from build123d import *

# Parameters (mm, degrees)
F0_W     = 76.2
F0_H     = 101.6
F1_DEPTH = 50.8
F2_W     = 101.6
F2_H     = 330
F3_DEPTH = 12.7
F4_W     = 101.6
F4_H     = 10
F5_DEPTH = 25.4
F6_W     = 63.5
F6_H     = 88.9
F7_DEPTH = 44.45
F9_DEPTH = 114.808


with BuildPart() as f1:
    # F0 (on Top) → F1 (new body)
    with BuildSketch(Plane.XY):
        Rectangle(F0_W, F0_H)
    extrude(amount=F1_DEPTH)

    # F2 (on face) → F3 (join)
    with BuildSketch(Plane.YZ.offset(38.1)):
        with Locations((0, 165)):
            Rectangle(F2_W, F2_H)
    extrude(amount=-F3_DEPTH)

    # F4 (on face) → F5 (join)
    with BuildSketch(Plane.YZ.offset(38.1)):
        with Locations((0, 325)):
            Rectangle(F4_W, F4_H)
        with Locations((0, 213.4)):
            Rectangle(F4_W, F4_H)
    extrude(amount=F5_DEPTH)

    # F6 (on face) → F7 (cut)
    with BuildSketch(Plane(origin=(0, 0, 0), x_dir=(1, 0, 0), z_dir=(0, 0, -1))):
        Rectangle(F6_W, F6_H)
    extrude(amount=-F7_DEPTH, mode=Mode.SUBTRACT)

    # F8 (on face) → F9 (cut)
    with BuildSketch(Plane.XZ.offset(50.8)):
        with BuildLine():
            ThreePointArc((-27.784303, 0), (-5.013912, -1.01281), (6.673748, 18.555406))
            ThreePointArc((6.673748, 18.555406), (0.164196, 34.270854), (-15.551252, 40.780406))
            ThreePointArc((-15.551252, 40.780406), (-36.839095, 24.9412), (-27.784303, 0))
        make_face()
        with BuildLine():
            ThreePointArc((-27.784303, 0), (-36.839095, 24.9412), (-15.551252, 40.780406))
            Line((-15.551252, 40.780406), (-38.1, 40.780406))
            Line((-38.1, 40.780406), (-38.1, 0))
            Line((-38.1, 0), (-27.784303, 0))
        make_face()
    extrude(amount=-F9_DEPTH, mode=Mode.SUBTRACT)


solid = f1.part
The model under review builds one solid part; all positions refer to its coordinate system, in mm. A direction names the side the tool comes from. Round coordinates to 2 decimals unless told otherwise and drop trailing zeros. Loops run counter-clockwise (first coordinate to the right, second up) from the corner with the lowest first, then second, coordinate; pieces in that order, holes last. Notation, with made-up numbers: (51.25, 73) -> (78.25, 73) arc R18 ccw to (78.25, 96) -> close; hole circle Ø8 at (-14, 55.25). An arc over 180 degrees is marked (long way). Return JSON: item names as keys, results as strings.
(1) Add section A-A on x = 45.5. Write out the cut boundary in (y, z), plus the area to 3 significant figures.
Solved:
{"outline": "(-50.8, 208.4) -> (50.8, 208.4) -> (50.8, 218.4) -> (-50.8, 218.4) -> close; (-50.8, 320) -> (50.8, 320) -> (50.8, 330) -> (-50.8, 330) -> close", "area": "2,030 mm2"}
(2) The part is to be moulded in two halves that separate along Z. For faces 1 (the flat face through (28, 50.8, 140)), 2 (the flat face through (38.1, -1, 268)), 3 (the flat face through (-33, -4, 40.78)), 4 (the flat face through (-7, 1, 50.8)), say which applies: released by +Z, released by -Z, zero draft, split by the parting line, or undercut.
Solved:
{"face 1": "zero draft", "face 2": "undercut", "face 3": "released by -Z", "face 4": "released by +Z"}
(3) Add section D-D on z = 215. Write out the cut boundary in (x, y).
Solved:
{"outline": "(25.4, -50.8) -> (63.5, -50.8) -> (63.5, 50.8) -> (25.4, 50.8) -> close"}
(4) For pin 1 (22 mm diameter, centred on y = 15, z = 23.5, fed in from -X); pin 2 (4 mm diameter, centred on y = -1.5, z = 205, fed in from -X); pin 3 (4 mm diameter, centred on y = -15, z = 43.5, fed in from +X), all flat-tipped, find the tip position at first contact; note any pin that passes through.
Solved:
{"pin 1": "x = 31.75", "pin 2": "x = 25.4", "pin 3": "x = 38.1"}
(5) For line 1 (Z direction, x = 47, y = -32.5); line 2 (X direction, y = 22, z = 208); line 3 (Y direction, x = 24.5, z = 29), list the stretches that pass through material, from the lowest coordinate up.
Solved:
{"line 1": "208.4 to 218.4, 320 to 330", "line 2": "25.4 to 38.1", "line 3": "-50.8 to -44.45, 44.45 to 50.8"}
(6) Add section B-B on x = -27. Write out the cut boundary in (y, z).
Solved:
{"outline": "(-50.8, 40.78) -> (-44.45, 40.78) -> (-44.45, 44.45) -> (44.45, 44.45) -> (44.45, 40.78) -> (50.8, 40.78) -> (50.8, 50.8) -> (-50.8, 50.8) -> close"}
(7) For faces 5 (the flat face through (28, -50.8, 140)), 6 (the flat face through (25.4, -1, 192)), 7 (the flat face through (14, -44.45, 22)), 8 (the flat face through (51, -1, 218.4)), 9 (the flat face through (38.1, -1, 103)), list the 3-axis set-ups (+Z, -Z, +X, -X, +Y, -Y) from which the entire face can be reached by the end or side of a thin tool; tool diameter is ignored.
Solved:
{"face 5": "+Z, -Z, +X, -X, -Y", "face 6": "+Z, -X, +Y, -Y", "face 7": "-Z", "face 8": "+X, +Y, -Y", "face 9": "-Z, +X, +Y, -Y"}
(8) Add section C-C on y = 23. Write out the cut boundary in (x, z).
Solved:
{"outline": "(-38.1, 40.78) -> (-31.75, 40.78) -> (-31.75, 44.45) -> (31.75, 44.45) -> (31.75, 0) -> (38.1, 0) -> (38.1, 208.4) -> (63.5, 208.4) -> (63.5, 218.4) -> (38.1, 218.4) -> (38.1, 320) -> (63.5, 320) -> (63.5, 330) -> (25.4, 330) -> (25.4, 50.8) -> (-38.1, 50.8) -> close"}
